Autodesk Inventor part; units mm, degrees
sketch "Sketch1" plane through (0, 0, 0) normal (0, 1, 0) x (-1, 0, 0)
  circle A0 centre (0, 0) radius 7
  line L0 (0, 0) -> (-31.25, 0)
  line L1 (-31.25, 0) -> (-31.25, -10)
  line L2 (-31.25, 0) -> (-31.25, 10)
  line L3 (-31.25, -10) -> (-1.4018, -13.1756)
  line L4 (-31.25, 10) -> (-1.4018, 13.1756)
  line L5 (0, 0) -> (38.25, 0)
  line L6 (38.25, 0) -> (38.25, -10)
  line L7 (38.25, -10) -> (1.1388, -13.1756)
  line L8 (38.25, 0) -> (38.25, 10)
  line L9 (38.25, 10) -> (1.4018, 13.1756)
  line L10 (-31.25, 0) -> (-28.25, 0)
  line L11 (-28.25, 0) -> (-28.25, -6.75)
  line L12 (-28.25, 0) -> (-28.25, 6.75)
  circle A1 centre (-28.25, -6.75) radius 2.25
  circle A2 centre (-28.25, 6.75) radius 2.25
  line L13 (38.25, 0) -> (35.25, 0)
  line L14 (35.25, 0) -> (35.25, -6.75)
  line L15 (35.25, 0) -> (35.25, 6.75)
  circle A3 centre (35.25, -6.75) radius 2.25
  circle A4 centre (35.25, 6.75) radius 2.25
  line L16 (1.1388, -13.1756) -> (-1.4018, -13.1756)
  line L17 (1.4018, 13.1756) -> (-1.4018, 13.1756)
  dimension "d2" = 14
  dimension "d3" = 31.25
  dimension "d4" = 10
  dimension "d5" = 10
  dimension "d6" = 38.25
  dimension "d7" = 10
  dimension "d8" = 10
  dimension "d9" = 3
  dimension "d10" = 6.75
  dimension "d11" = 6.75
  dimension "d12" = 4.5
  dimension "d13" = 4.5
  dimension "d14" = 3
  dimension "d15" = 6.75
  dimension "d16" = 6.75
  dimension "d17" = 4.5
  dimension "d18" = 4.5
extrude "Extrusion1" add sketch "Sketch1" along normal blind 4.5 contours L5 L6 L7 L16 L3 L1 L0 A0 | A0 L0 L2 L4 L17 L9 L8 L5
sketch "Sketch2" plane through (0, 0, 0) normal (0, 1, 0) x (-1, 0, 0)
  circle A0 centre (0, 0) radius 13.25
  circle A1 centre (0, 0) radius 11.25
  dimension "d21" = 26.5
  dimension "d22" = 22.5
extrude "Extrusion2" add sketch "Sketch2" along normal blind 11
fillet "Fillet1" radius 3 1 edges at (-38.25, 2.25, -10)
fillet "Fillet2" radius 3 3 edges at (-38.25, 2.25, 10) (31.25, 2.25, 10) (31.25, 2.25, -10)
properties part number "bearing_holder"
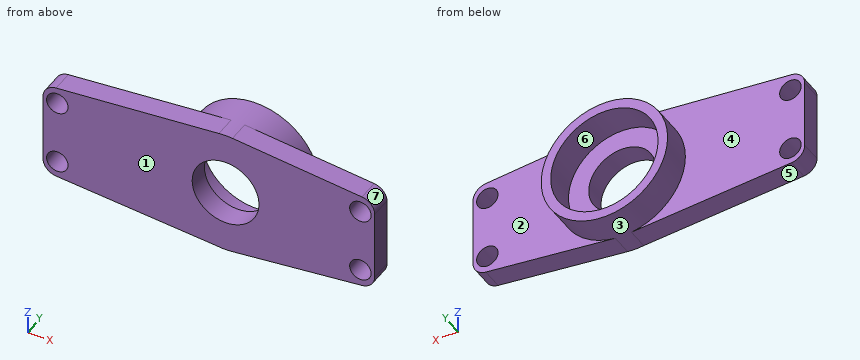
Verification items for the finished model (mm, model axes). Face numbers are marked on the shaded views. A direction names the side the tool comes from. Give positions to 0.01 mm unless a question says otherwise; leave off trailing zeros. Loops run counter-clockwise (first coordinate to the right, second up) from the corner with the lowest first, then second, coordinate; pieces in that order, holes last.
1) Draft check along X on the marked faces 4, 5, 6 and 7. Enter one of: pulls with the +X half, pulls with the -X half, needs draft (parallel to the pull), parting line crosses it, or undercut.
2) Depth check by flat-ended pin: pin 1 Ø7 at (x, z) = (2.5, 3.5) entering from +Y; pin 2 Ø1.5 at (x, y) = (5, 3) entering from -Z. Enter the tip coordinate at first touch or a pass-through.
3) Set-up check for the marked faces 1, 2 and 3: record each of +Z, -Z, +X, -X, +Y, -Y from which the full face is reachable in a straight line by a thin tool's end or side.
4) Sectioned sample at D-D, the plane y = 9.5. Enter the section's corners in (x, z), then the cut area to 3 significant figures.
5) Sectioned sample at B-B, the plane z = -3. Enter the section's corners in (x, y), then the cut area to 3 significant figures.
6) Sectioned sample at C-C, the plane z = -8.25. Enter the section's corners in (x, y).
7) Thickness scan on line 1 along X through (y, z) = (1.55, 0); line 2 along Z through (x, y) = (27, 4); line 3 along Y through (x, z) = (-26.5, -6). Record the ranges inside material, lowest first.
8) Sectioned sample at A-A, the plane x = 0. Enter the section's corners in (y, z).
Answers:
1. face 4: needs draft
1. face 5: pulls with the -X half
1. face 6: undercut
1. face 7: pulls with the +X half
2. pin 1: stops at y = 4.5
2. pin 2: stops at z = -12.87
3. face 1: +Z, -Z, +X, -X, -Y
3. face 2: +X, +Y
3. face 3: +Y
4. outline: circle Ø26.5 at (0, 0); hole circle Ø22.5 at (0, 0)
4. area: 154 mm2
5. outline: (-38.25, 0) - (-6.32, 0) - (-6.32, 4.5) - (-10.84, 4.5) - (-10.84, 11) - (-12.91, 11) - (-12.91, 4.5) - (-38.25, 4.5) - close; (6.32, 0) - (31.25, 0) - (31.25, 4.5) - (12.91, 4.5) - (12.91, 11) - (10.84, 11) - (10.84, 4.5) - (6.32, 4.5) - close
5. area: 283 mm2
6. outline: (-38.08, 0) - (-36.93, 0) - (-36.93, 4.5) - (-38.08, 4.5) - close; (-33.57, 0) - (26.57, 0) - (26.57, 4.5) - (10.37, 4.5) - (10.37, 11) - (7.65, 11) - (7.65, 4.5) - (-7.65, 4.5) - (-7.65, 11) - (-10.37, 11) - (-10.37, 4.5) - (-33.57, 4.5) - close; (29.93, 0) - (31.1, 0) - (31.1, 4.5) - (29.93, 4.5) - close
7. line 1: x = -38.25 to -7, 7 to 31.25
7. line 2: z = -10.45 to -8.62, -4.88 to 4.88, 8.62 to 10.45
7. line 3: y = 0 to 4.5
8. outline: (0, -13.25) - (11, -13.25) - (11, -11.25) - (4.5, -11.25) - (4.5, -7) - (0, -7) - close; (0, 7) - (4.5, 7) - (4.5, 11.25) - (11, 11.25) - (11, 13.25) - (0, 13.25) - close
